For this review, take the finished solid that the model builds, in its own axes (mm). A direction names the side the tool comes from. Give positions to 0.01 mm unless a question says otherwise; leave off trailing zeros. Order: outer loops, then holes, each group sorted by start corner. A loop starts at its lowest first (then second) coordinate and runs counter-clockwise, first axis right, second up. Notation, with made-up numbers: (49, 43.25) - (63, 43.25) arc R15 cw to (63, 53.25) - close; hole circle Ø4 at (75, 40.5). An arc over 180 degrees is marked (long way). Put each result on its own line as item: value. Start each with the question number.
```python
from build123d import *

# Parameters (mm, degrees)
F0_W     = 127
F0_H     = 127
F1_DEPTH = 127
F2_SIZE  = 25.4
F3_R     = 25.4
F4_DEPTH = 610.6993397


# Not quite as in the source:
# - an extrude ends at something that could not be found from the text; its depth is read off the source's solid
# - a feature of the source that left no trace in its solid (it failed there, or was rolled back) is left out


with BuildPart() as f1:
    # F0 (on Front) → F1 (new body)
    with BuildSketch(Plane.XZ):
        with Locations((0, -1.5167773236)):
            Rectangle(F0_W, F0_H)
    extrude(amount=F1_DEPTH)

    # F2
    f2_edges = [f1.edges().sort_by_distance(p)[0] for p in [
        (-63.5, -63.5, 61.983223),
        (63.5, -63.5, 61.983223),
    ]]
    chamfer(f2_edges, length=F2_SIZE)

    # F3 (on face) → F4 (join, through all)
    with BuildSketch(Plane.XZ.offset(127)):
        Circle(F3_R)
    extrude(amount=F4_DEPTH)


solid = f1.part
```
1. Wall thickness on line 1 (Y direction, x = 3, z = 28); line 2 (Z direction, x = -19.5, y = -472.5); line 3 (Z direction, x = -11.5, y = -619.5): over which ranges is each line inside the solid? List them lowest first. Write a range as from..to.
2. Add section B-B, the plane y = -110.5. Give the boundary of the cut face in (x, z).
3. Tool access review of faces 1 (the face through (0, -737.699, 0)), 2 (the face through (-1, -127, -29)): name each direction out of +Z, -Z, +X, -X, +Y, -Y from which nothing blocks a thin tool from reaching the whole face with its end or side.
4. Add section D-D, the plane y = -327.5. Give the boundary of the cut face in (x, z), then the cut area to 3 significant figures.
5. Clearance check with flat-ended pins moving along their axes: pin 1 (8 mm diameter, centred on x = 7.5, z = 16, fed in from +Y); pin 2 (8 mm diameter, centred on x = 10, y = -184.5, fed in from +Z); pin 3 (2 mm diameter, centred on y = -453, z = 18, fed in from +X); pin 4 (6 mm diameter, centred on y = -275.5, z = -2.5, fed in from +X). State where each tip first meets the part, or that it passes through.
6. Add section C-C, the plane z = 0. Give the boundary of the cut face in (x, y), then the cut area to 3 significant figures.
7. Add section A-A, the plane x = 0. Give the boundary of the cut face in (y, z).
Found:
1. line 1: y = -127..0
1. line 2: z = -16.28..16.28
1. line 3: z = -22.65..22.65
2. outline: (-63.5, -65.02) - (63.5, -65.02) - (63.5, 36.58) - (38.1, 61.98) - (-38.1, 61.98) - (-63.5, 36.58) - close
3. face 1: +Z, -Z, +X, -X, -Y
3. face 2: -Y
4. outline: circle Ø50.8 at (0, 0)
4. area: 2,030 mm^2
5. pin 1: stops at y = 0
5. pin 2: stops at z = 24.68
5. pin 3: stops at x = 18.87
5. pin 4: stops at x = 25.4
6. outline: (-63.5, -127) - (-25.4, -127) - (-25.4, -737.7) - (25.4, -737.7) - (25.4, -127) - (63.5, -127) - (63.5, 0) - (-63.5, 0) - close
6. area: 47,200 mm^2
7. outline: (-737.7, -25.4) - (-127, -25.4) - (-127, -65.02) - (0, -65.02) - (0, 61.98) - (-127, 61.98) - (-127, 25.4) - (-737.7, 25.4) - close
